```python
from build123d import *

# Parameters (mm, degrees)
SKETCH1_R           = 12.5
BOSS_EXTRUDE1_DEPTH = 50
FILLET1_R           = 25
SKETCH2_R           = 10
SKETCH2_W           = 50
SKETCH2_H           = 20
CUT_EXTRUDE1_DEPTH  = 55


with BuildPart() as part:
    # Sketch1 → Boss-Extrude1 (new body)
    with BuildSketch(Plane.XY):
        with BuildLine():
            ThreePointArc((0, 50), (-25, 25), (0, 0))
            Line((0, 0), (125, 0))
            Line((125, 0), (125, 15))
            Line((125, 15), (75, 15))
            Line((75, 15), (75, 35))
            Line((75, 35), (125, 35))
            Line((125, 35), (125, 50))
            Line((125, 50), (0, 50))
        make_face()
        with Locations((0, 25)):
            Circle(SKETCH1_R, mode=Mode.SUBTRACT)
    extrude(amount=BOSS_EXTRUDE1_DEPTH)

    # Fillet1
    fillet1_edges = [part.edges().sort_by_distance(p)[0] for p in [
        (125, 7.5, 0),
        (125, 42.5, 0),
        (125, 7.5, 50),
        (125, 42.5, 50),
    ]]
    fillet(fillet1_edges, radius=FILLET1_R - 0.0001)  # a hair under: the kernel refuses the full size

    # Sketch2 → Cut-Extrude1 (cut)
    with BuildSketch(Plane(origin=(0, 50, 0), x_dir=(1, 0, 0), z_dir=(0, 1, 0))):
        with Locations(Location((100, -25, 0), (0, 0, 270))):
            Circle(SKETCH2_R)
        with Locations((0, -25)):
            Rectangle(SKETCH2_W, SKETCH2_H)
    extrude(amount=-CUT_EXTRUDE1_DEPTH, mode=Mode.SUBTRACT)


solid = part.part
```
Source: CAD feature listing. Evaluate the final solid. Frame: model axes, mm. A direction names the side the tool comes from. Give positions to 0.01 mm unless a question says otherwise; leave off trailing zeros. Write each loop counter-clockwise with the first axis right and the second up, starting at its lowest first coordinate (ties: lowest second). Pieces come first, ordered by that corner, then holes. Notation, with made-up numbers: (76, -20) - (98, -20) arc R19 cw to (98, -6) - close; hole circle Ø3 at (-22.5, 38). An arc over 180 degrees is marked (long way). One line per item, written item: value. Start each with the question number.
Q1. Section query A-A, the plane x = 78. Return the cut outline in (y, z).
Q2. Section query D-D, the plane x = 1.5. Return the cut outline in (y, z), then the cut area to 3 significant figures.
Q3. First-contact query: pin 1 Ø1.5 at (y, z) = (44.5, 39.5) entering from +X; pin 2 Ø8 at (y, z) = (9.5, 18) entering from -X; pin 3 Ø22 at (y, z) = (17.5, 20.5) entering from -X. Flat tips, straight axial feed; report the tip coordinate or a pass-through.
Q4. Set-up query: faces 5 (the face through (63, 50, 25)), 6 (the face through (89, 35, 25)), 7 (the face through (25, 25, 25)). Return all of +Z, -Z, +X, -X, +Y, -Y with unobstructed straight access to the full face (end or side cutting, diameter ignored); none if empty.
Q5. Draft query along Z for faces 1 (the face through (117.871, 7.605, 42.482)), 2 (the face through (108.43, 42.6, 30.38)), 3 (the face through (-24.994, 25.55, 42.395)), 4 (the face through (16, 25, 35)). Return one class per face: +Z half, -Z half, draft (parallel to the pull), parting line (faces both ways), or undercut.
Q6. Material intervals for probe 1 along Y at (x, z) = (0, 7.25); probe 2 along Z at (x, y) = (10, 37); probe 3 along X at (y, z) = (9.75, 25), sorted ascending. Write a range as from..to.
Q7. Section query B-B, the plane y = 25. Return the cut outline in (x, z).
Q8. Section query C-C, the plane z = 17.5. Return the cut outline in (x, y).
Answer:
1. outline: (0, 0) - (15, 0) - (15, 50) - (0, 50) - close; (35, 0) - (50, 0) - (50, 50) - (35, 50) - close
2. outline: (0, 0) - (12.59, 0) - (12.59, 15) - (0, 15) - close; (0, 35) - (12.59, 35) - (12.59, 50) - (0, 50) - close; (37.41, 0) - (50, 0) - (50, 15) - (37.41, 15) - close; (37.41, 35) - (50, 35) - (50, 50) - (37.41, 50) - close
2. area: 755 mm2
3. pin 1: stops at x = 120.88
3. pin 2: stops at x = -21.44
3. pin 3: stops at x = -25
4. face 5: +Z, -Z, +X, -X, +Y
4. face 6: +Z, -Z, +X
4. face 7: -X, +Y, -Y
5. face 1: +Z half
5. face 2: undercut
5. face 3: draft
5. face 4: undercut
6. probe 1: y = 0..12.5, 37.5..50
6. probe 2: z = 0..15, 35..50
6. probe 3: x = 25..90, 110..125
7. outline: (-25, 0) - (-12.5, 0) - (-12.5, 15) - (-25, 15) - close; (-25, 35) - (-12.5, 35) - (-12.5, 50) - (-25, 50) - close; (12.5, 0) - (75, 0) - (75, 50) - (12.5, 50) - (12.5, 35) - (25, 35) - (25, 15) - (12.5, 15) - close
8. outline: (25, 0) - (93.39, 0) - (93.39, 15) - (75, 15) - (75, 35) - (93.39, 35) - (93.39, 50) - (25, 50) - close; (106.61, 0) - (123.85, 0) - (123.85, 15) - (106.61, 15) - close; (106.61, 35) - (123.85, 35) - (123.85, 50) - (106.61, 50) - close
